Here's how the part is built. I have some questions about the finished solid (model axes, mm). Face numbers are marked on the shaded views. Round coordinates to 2 decimals unless told otherwise and drop trailing zeros. Loops run counter-clockwise (first coordinate to the right, second up) from the corner with the lowest first, then second, coordinate; pieces in that order, holes last. Notation, with made-up numbers: (61.5, -23.75) - (120.5, -23.75) arc R19 ccw to (120.5, -5.75) - close; hole circle Ø11 at (-29, 65.25). An arc over 180 degrees is marked (long way). Answer as a JSON object with one key per item and string values. Group by question number.
1) Will this pin go through, and if not, where does the flat tip stop? P1, Ø3, axis at y = -3.11, z = 4, coming from the +X side.
2) If we mould it in two halves opening along X, with no side actions, what happens to the marked faces 1, 2 and 3? For each: pulls with the +X half, pulls with the -X half, needs draft (parallel to the pull), parting line crosses it, or undercut.
3) I want a section at B-B, the plane x = 21. Please give me the cut outline in (y, z), then the cut area to 3 significant figures.
4) If I drill on line 1 along Y through (x, z) = (31, 4); line 2 along Y through (x, z) = (16, 5.5); line 3 along Z through (x, y) = (21.5, -3.25), over which ranges is the centre line in solid material (lowest first)? Write a range as [from, to].
5) I want a section at A-A, the plane z = 4. Please give me the cut outline in (x, y), then the cut area to 3 significant figures.
from build123d import *

# Parameters (mm, degrees)
SKETCH_1_W          = 39.1
SKETCH_1_H          = 30
EXTRUDE_1_DEPTH     = 8
SKETCH_2_R          = 1.8
CUT_EXTRUDE_1_DEPTH = 44.826627362


with BuildPart() as part:
    # 草圖1 → 填料-伸長1 (new body)
    with BuildSketch(Plane.XY):
        with Locations((15.847455636, -3.109756098)):
            Rectangle(SKETCH_1_W, SKETCH_1_H)
    extrude(amount=EXTRUDE_1_DEPTH)

    # 草圖2 → 除料-伸長1 (cut, through all)
    with BuildSketch(Plane.ZY.offset(3.702544364)):
        with Locations((4, 4.890243902)):
            Circle(SKETCH_2_R)
        with Locations((4, -3.109756098)):
            Circle(SKETCH_2_R)
        with Locations((4, -11.109756098)):
            Circle(SKETCH_2_R)
    extrude(amount=-CUT_EXTRUDE_1_DEPTH, mode=Mode.SUBTRACT)


solid = part.part
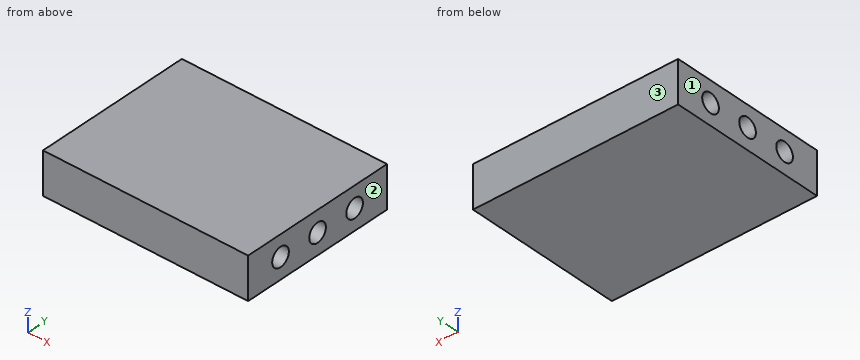
Outcome:
{
 "1": {"P1": "through"},
 "2": {"face 1": "pulls with the -X half", "face 2": "pulls with the +X half", "face 3": "needs draft"},
 "3": {"outline": "(-18.11, 0) - (11.89, 0) - (11.89, 8) - (-18.11, 8) - close; hole circle Ø3.6 at (-11.11, 4); hole circle Ø3.6 at (-3.11, 4); hole circle Ø3.6 at (4.89, 4)", "area": "209 mm^2"},
 "4": {"line 1": "[-18.11, -12.91], [-9.31, -4.91], [-1.31, 3.09], [6.69, 11.89]", "line 2": "[-18.11, -12.1], [-10.11, -4.1], [-2.11, 3.9], [5.89, 11.89]", "line 3": "[0, 2.21], [5.79, 8]"},
 "5": {"outline": "(-3.7, -18.11) - (35.4, -18.11) - (35.4, -12.91) - (-3.7, -12.91) - close; (-3.7, -9.31) - (35.4, -9.31) - (35.4, -4.91) - (-3.7, -4.91) - close; (-3.7, -1.31) - (35.4, -1.31) - (35.4, 3.09) - (-3.7, 3.09) - close; (-3.7, 6.69) - (35.4, 6.69) - (35.4, 11.89) - (-3.7, 11.89) - close", "area": "751 mm^2"}
}
